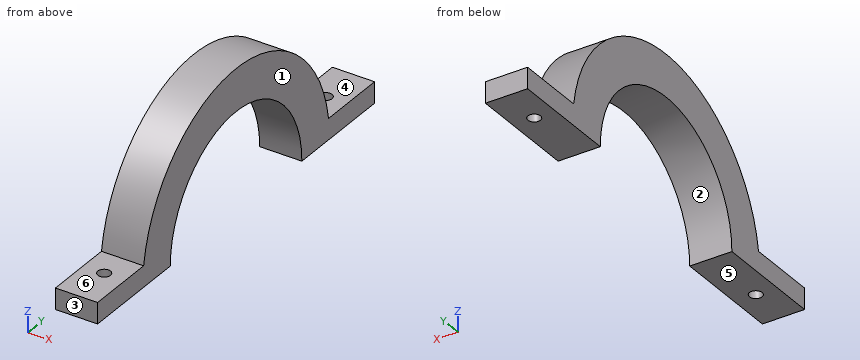
```python
from build123d import *

# Parameters (mm, degrees)
F1_DEPTH = 10
F2_R     = 1.5
F3_DEPTH = 25


with BuildPart() as f1:
    # F0 (on Right) → F1 (new body)
    with BuildSketch(Plane.YZ):
        with BuildLine():
            Line((-50, 0), (-23.75, 0))
            ThreePointArc((-23.75, 0), (0, 23.75), (23.75, 0))
            Line((23.75, 0), (50, 0))
            Line((50, 0), (50, 5))
            Line((50, 5), (33.377575, 5))
            ThreePointArc((33.377575, 5), (0, 33.75), (-33.377575, 5))
            Line((-33.377575, 5), (-50, 5))
            Line((-50, 5), (-50, 0))
        make_face()
    extrude(amount=F1_DEPTH)

    # F2 (on face) → F3 (cut)
    with BuildSketch(Plane.XY.offset(5)):
        with Locations((5, 40)):
            Circle(F2_R)
        with Locations((5, -40)):
            Circle(F2_R)
    extrude(amount=-F3_DEPTH, mode=Mode.SUBTRACT)


solid = f1.part
```
Model file for the job. Use its own axes, mm. Face numbers are marked on the shaded views. A direction names the side the tool comes from. Round coordinates to 2 decimals unless told otherwise and drop trailing zeros. Write each loop counter-clockwise with the first axis right and the second up, starting at its lowest first coordinate (ties: lowest second). Pieces come first, ordered by that corner, then holes. Notation, with made-up numbers: M 69.25,74.25 L 107.25,74.25 A26 ccw 107.25,108.25 Z; hole C 14.5,8 d11. An arc over 180 degrees is marked long. Put each result on its own line as item: value.
Item 1: Cut at B-B (y = -40). List the corners of the cut face in (x, z), and give its area (3 significant figures).
Responses:
outline: M 0,0 L 3.5,0 L 3.5,5 L 0,5 Z; M 6.5,0 L 10,0 L 10,5 L 6.5,5 Z
area: 35.0 mm²
Item 2: Cut at A-A (x = 5). List the corners of the cut face in (y, z).
Responses:
outline: M -50,0 L -41.5,0 L -41.5,5 L -50,5 Z; M -38.5,0 L -23.75,0 A23.75 cw 23.75,0 L 38.5,0 L 38.5,5 L 33.38,5 A33.75 ccw -33.38,5 L -38.5,5 Z; M 41.5,0 L 50,0 L 50,5 L 41.5,5 Z
Item 3: Cut at D-D (z = 7). List the corners of the cut face in (x, y).
Responses:
outline: M 0,-33.02 L 10,-33.02 L 10,-22.69 L 0,-22.69 Z; M 0,22.69 L 10,22.69 L 10,33.02 L 0,33.02 Z
Item 4: Mould opens along Y. For the marked faces 1, 2 and 3 say: +Y half, -Y half, draft (parallel to the pull), parting line (faces both ways), or undercut.
Responses:
face 1: draft
face 2: undercut
face 3: -Y half
Item 5: Flat gauge pins, fed straight in: P1, Ø5, axis at x = 2.5, y = 45, coming from the +Z side; P2, Ø2, axis at x = 6, y = -18.5, coming from the -Z side; P3, Ø5, axis at x = 8.5, y = -14, coming from the -Z side. Where does each tip first touch, or does it go through?
Responses:
P1: z = 5
P2: z = 13.56
P3: z = 17.08
Item 6: Tool access for the marked faces 4, 5 and 6: list every direction of +Z, -Z, +X, -X, +Y, -Y with a clear straight run to the whole face (end or side of a thin tool).
Responses:
face 4: +Z, +X, -X, +Y
face 5: -Z, +X, -X, +Y, -Y
face 6: +Z, +X, -X, -Y
Item 7: Cut at C-C (z = 3). List the corners of the cut face in (x, y), and give its area (3 significant figures).
Responses:
outline: M 0,-50 L 10,-50 L 10,-23.56 L 0,-23.56 Z; M 0,23.56 L 10,23.56 L 10,50 L 0,50 Z; hole C 5,-40 d3; hole C 5,40 d3
area: 515 mm²
Item 8: Probe L1, parallel to Y at x = 5, z = 1.85; L2, parallel to Y at x = 2, z = 10; L3, parallel to Y at x = 7, z = 16. List the from-to ranges inside material, lowest first. Write a range as from..to.
Responses:
L1: -50..-41.5, -38.5..-23.68, 23.68..38.5, 41.5..50
L2: -32.23..-21.54, 21.54..32.23
L3: -29.72..-17.55, 17.55..29.72
